Design review of the part built by this model. Coordinates are the model's own, in mm. A direction names the side the tool comes from. Give positions to 0.01 mm unless a question says otherwise; leave off trailing zeros. Write each loop counter-clockwise with the first axis right and the second up, starting at its lowest first coordinate (ties: lowest second). Pieces come first, ordered by that corner, then holes. Notation, with made-up numbers: (85, -18) - (134, -18) arc R26 ccw to (134, -2) - close; hole circle Ø4 at (-2, -26). An arc over 180 degrees is marked (long way). Use a Markdown table: item, result. Add a question column.
```python
from build123d import *

# Parameters (mm, degrees)
F0_R = 0.889


with BuildPart() as f2:
    # F2: sweep along a path in F1
    with BuildLine(Plane.YZ) as f2_path:
        Line((0, 0), (-8.89, 0))
        Line((-8.89, 0), (-8.89, 25.4))
        Line((-8.89, 25.4), (8.3446010148, 25.4))
        Line((8.3446010148, 25.4), (8.3446010148, 0))
        Line((8.3446010148, 0), (1.5816572689, 0))
    # F0 (on Front) → F2 (sweep)
    with BuildSketch(Plane.XZ):
        Circle(F0_R)
    sweep(path=f2_path.line, transition=Transition.RIGHT)


solid = f2.part
```
(1) Add section D-D (z = 25.4). State the section outline as (x, y) points.
(2) Tool access review of faces 3 (the face through (0, 1.582, 0)), 4 (the face through (-0.19, -4.96, -0.87)): name each direction out of +Z, -Z, +X, -X, +Y, -Y from which nothing blocks a thin tool from reaching the whole face with its end or side.
(3) Mouldability with a two-part tool opening along Z and no side actions: class faces 1 (the face through (0, 0, 0)), 2 (the face through (0.41, -0.14, 26.19)) as +Z half, -Z half, draft (parallel to the pull), parting line (faces both ways), or undercut.
(4) Add section B-B (z = 0). State the section outline as (x, y) points, and give its area (3 significant figures).
(5) Insertion check: pin 1 (0.5 mm diameter, centred on x = 0.5, z = 0, fed in from -Y). The pin has a flat end and moves straight along its axis. Give the tip position at first contact, or say it passes through.
(6) For line 1 along Z through (x, y) = (0.1, -2); line 2 along Y through (x, z) = (-0.1, 8.5); line 3 along Z through (x, y) = (-0.35, 3), list the stretches that pass through material, from the lowest coordinate up.
(7) Add section A-A (x = 0). State the section outline as (y, z) points, and give its area (3 significant figures).
(8) Add section C-C (y = 5.5). State the section outline as (x, z) points, and give its area (3 significant figures).
Answers follow:
| question | item | result |
|---|---|---|
| 1 | outline | (-0.89, -8.89) arc R0.89 ccw to (0.89, -8.89) - (0.89, 8.34) arc R0.89 ccw to (-0.89, 8.34) - close |
| 2 | face 3 | -Z, +X, -X |
| 2 | face 4 | none |
| 3 | face 1 | draft |
| 3 | face 2 | undercut |
| 4 | outline | (-0.89, -8.89) arc R0.89 ccw to (0.89, -8.89) - (0.89, 0) - (-0.89, 0) - close; (-0.89, 1.58) - (0.89, 1.58) - (0.89, 8.34) arc R0.89 ccw to (-0.89, 8.34) - close |
| 4 | area | 30.3 mm^2 |
| 5 | pin 1 | y = -9.74 |
| 6 | line 1 | -0.88 to 0.88, 24.52 to 26.28 |
| 6 | line 2 | -9.77 to -8.01, 7.46 to 9.23 |
| 6 | line 3 | -0.82 to 0.82, 24.58 to 26.22 |
| 7 | outline | (-9.78, -0.89) - (0, -0.89) - (0, 0.89) - (-8, 0.89) - (-8, 24.51) - (7.46, 24.51) - (7.46, 0.89) - (1.58, 0.89) - (1.58, -0.89) - (9.23, -0.89) - (9.23, 26.29) - (-9.78, 26.29) - close |
| 7 | area | 149 mm^2 |
| 8 | outline | circle Ø1.78 at (0, 0); circle Ø1.78 at (0, 25.4) |
| 8 | area | 4.97 mm^2 |
